Check sheet for the drawn part. Datum: minimum x, y, z corner. Units: mm. Round coordinates to 2 decimals unless told otherwise and drop trailing zeros. Write each loop counter-clockwise with the first axis right and the second up, starting at its lowest first coordinate (ties: lowest second). Pieces come first, ordered by that corner, then holes.
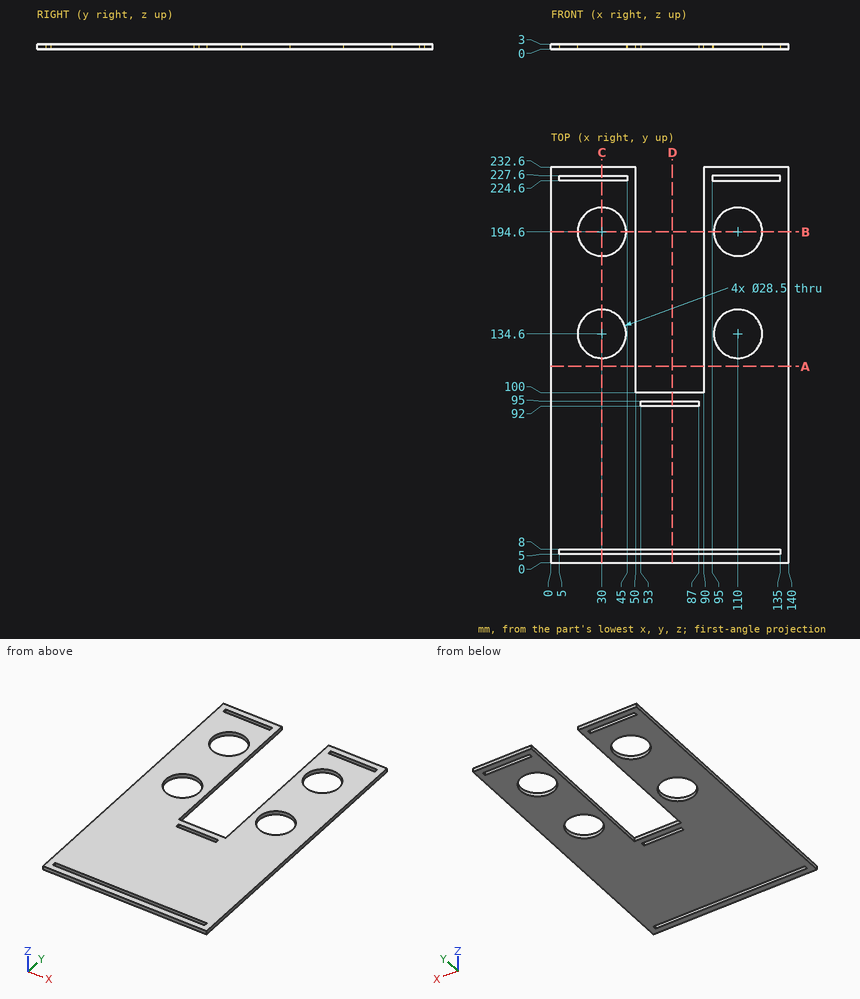
1. Go/stop test with flat-tipped pins: pin 1 (1.5 mm diameter, centred on x = 72, z = 2, fed in from +Y); pin 2 (1.5 mm diameter, centred on x = 19.5, z = 1, fed in from -Y). Record where each tip stops, or that it passes through.
2. Sectioned sample at A-A, the plane y = 115.5. Enter the section's corners in (x, z), plus the area to 3 significant figures.
3. Sectioned sample at C-C, the plane x = 30. Enter the section's corners in (y, z).
4. Sectioned sample at D-D, the plane x = 71.5. Enter the section's corners in (y, z), plus the area to 3 significant figures.
5. Sectioned sample at B-B, the plane y = 194.6. Enter the section's corners in (x, z).
6. Scan lines: line 1 along Y through (x, z) = (110, 1.8); line 2 along Y through (x, z) = (127, 1.15); line 3 along Y through (x, z) = (80.5, 2.55). Record each from-to range of solid material in increasing order.
Computed values:
1. pin 1: stops at y = 100
1. pin 2: stops at y = 0
2. outline: (0, 0) - (50, 0) - (50, 3) - (0, 3) - close; (90, 0) - (140, 0) - (140, 3) - (90, 3) - close
2. area: 300 mm2
3. outline: (0, 0) - (5, 0) - (5, 3) - (0, 3) - close; (8, 0) - (120.35, 0) - (120.35, 3) - (8, 3) - close; (148.85, 0) - (180.35, 0) - (180.35, 3) - (148.85, 3) - close; (208.85, 0) - (224.6, 0) - (224.6, 3) - (208.85, 3) - close; (227.6, 0) - (232.6, 0) - (232.6, 3) - (227.6, 3) - close
4. outline: (0, 0) - (5, 0) - (5, 3) - (0, 3) - close; (8, 0) - (92, 0) - (92, 3) - (8, 3) - close; (95, 0) - (100, 0) - (100, 3) - (95, 3) - close
4. area: 282 mm2
5. outline: (0, 0) - (15.75, 0) - (15.75, 3) - (0, 3) - close; (44.25, 0) - (50, 0) - (50, 3) - (44.25, 3) - close; (90, 0) - (95.75, 0) - (95.75, 3) - (90, 3) - close; (124.25, 0) - (140, 0) - (140, 3) - (124.25, 3) - close
6. line 1: y = 0 to 5, 8 to 120.35, 148.85 to 180.35, 208.85 to 224.6, 227.6 to 232.6
6. line 2: y = 0 to 5, 8 to 224.6, 227.6 to 232.6
6. line 3: y = 0 to 5, 8 to 92, 95 to 100
